```python
from build123d import *

# Parameters (mm, degrees)
SKETCH1_W            = 40.5
SKETCH1_H            = 20
BOSS_EXTRUDE1_DEPTH  = 35.5
BOSS_EXTRUDE2_DEPTH  = 2
SKETCH3_R            = 6.4
BOSS_EXTRUDE3_DEPTH  = 1
SKETCH4_R            = 5.575
BOSS_EXTRUDE4_DEPTH  = 0.5
BOSS_EXTRUDE5_DEPTH  = 2.5
MIRROR2_COPY_1_DEPTH = 2.5


with BuildPart() as part:
    # Sketch1 → Boss-Extrude1 (new body)
    with BuildSketch(Plane(origin=(0, 0, 0), x_dir=(1, 0, 0), z_dir=(0, 1, 0))):
        Rectangle(SKETCH1_W, SKETCH1_H)
    extrude(amount=BOSS_EXTRUDE1_DEPTH)

    # Sketch2 → Boss-Extrude2 (add)
    with BuildSketch(Plane(origin=(0, 35.5, 0), x_dir=(1, 0, 0), z_dir=(0, 1, 0))):
        with BuildLine():
            Line((-5.75, -9), (14.25, -9))
            Line((14.25, -9), (14.25, -4.8))
            ThreePointArc((14.25, -4.8), (16.65, 0), (14.25, 4.8))
            Line((14.25, 4.8), (14.25, 9))
            Line((14.25, 9), (-5.75, 9))
            ThreePointArc((-5.75, 9), (-20.108898944, 0), (-5.75, -9))
        make_face()
    extrude(amount=BOSS_EXTRUDE2_DEPTH)

    # Sketch3 → Boss-Extrude3 (add)
    with BuildSketch(Plane(origin=(0, 37.5, 0), x_dir=(1, 0, 0), z_dir=(0, 1, 0))):
        with Locations(Location((-10.108898944, 0, 0), (0, 0, 270))):
            Circle(SKETCH3_R)
    extrude(amount=BOSS_EXTRUDE3_DEPTH)

    # Sketch4 → Boss-Extrude4 (add)
    with BuildSketch(Plane(origin=(0, 38.5, 0), x_dir=(1, 0, 0), z_dir=(0, 1, 0))):
        with Locations(Location((-10.108898944, 0, 0), (0, 0, 270))):
            Circle(SKETCH4_R)
    extrude(amount=BOSS_EXTRUDE4_DEPTH)

    # Sketch5 → Boss-Extrude5 (add)
    with BuildSketch(Plane(origin=(0, 29.5, 0), x_dir=(1, 0, 0), z_dir=(0, 1, 0))):
        with BuildLine():
            Line((20.25, 9), (27.25, 9))
            Line((27.25, 9), (27.25, 6.25))
            Line((27.25, 6.25), (26.177050983, 6.25))
            ThreePointArc((26.177050983, 6.25), (22.25, 4.75), (26.177050983, 3.25))
            Line((26.177050983, 3.25), (27.25, 3.25))
            Line((27.25, 3.25), (27.25, 0))
            Line((27.25, 0), (20.25, 0))
            Line((20.25, 0), (20.25, 9))
        make_face()
    boss_extrude5 = extrude(amount=-BOSS_EXTRUDE5_DEPTH)

    # Mirror1: Boss-Extrude5 across plane
    add(boss_extrude5.mirror(Plane(origin=(0, 0, 0), x_dir=(0, 0, 1), z_dir=(1, 0, 0))))

    # Mirror2: Boss-Extrude5 across plane
    add(boss_extrude5.mirror(Plane.XY))

    # Mirror2 copy 1 sketch → Mirror2 copy 1 (add)
    with BuildSketch(Plane(origin=(0, 29.5, 0), x_dir=(-1, 0, 0), z_dir=(0, 1, 0))):
        with BuildLine():
            Line((20.25, 9), (27.25, 9))
            Line((27.25, 9), (27.25, 6.25))
            Line((27.25, 6.25), (26.177050983, 6.25))
            ThreePointArc((26.177050983, 6.25), (22.25, 4.75), (26.177050983, 3.25))
            Line((26.177050983, 3.25), (27.25, 3.25))
            Line((27.25, 3.25), (27.25, 0))
            Line((27.25, 0), (20.25, 0))
            Line((20.25, 0), (20.25, 9))
        make_face()
    extrude(amount=-MIRROR2_COPY_1_DEPTH)


solid = part.part
```
For this review, take the finished solid that the model builds, in its own axes (mm). A direction names the side the tool comes from. Round coordinates to 2 decimals unless told otherwise and drop trailing zeros. Write each loop counter-clockwise with the first axis right and the second up, starting at its lowest first coordinate (ties: lowest second). Pieces come first, ordered by that corner, then holes. Notation, with made-up numbers: (-3, 6.5) - (21, 6.5) arc R12 ccw to (21, 10.5) - close; hole circle Ø11 at (55.25, -29.75). An arc over 180 degrees is marked (long way). Answer as a JSON object with one key per item and string values.
1. Tool access review of faces 5 (the face through (-27, 28, -6.25)), 6 (the face through (23, 27, 0)), 7 (the face through (-20.09, 35.5, 2.18)): name each direction out of +Z, -Z, +X, -X, +Y, -Y from which nothing blocks a thin tool from reaching the whole face with its end or side.
Response values:
{"face 5": "-X, +Y, -Y", "face 6": "+Z, -Z, +X, -Y", "face 7": "-X, +Y"}
2. Draft analysis for pull direction Z (two halves, no side actions). For faces 1 (the face through (-27, 28, -3.25)), 2 (the face through (23, 29.5, 0)), 3 (the face through (-24, 28, 9)), 4 (the face through (22.25, 28.27, 4.83)), state which applies: +Z half, -Z half, draft (parallel to the pull), parting line (faces both ways), or undercut.
Response values:
{"face 1": "undercut", "face 2": "draft", "face 3": "+Z half", "face 4": "undercut"}
3. We need section A-A on x = -24.5. Give the boundary of the cut face in (y, z).
Response values:
{"outline": "(27, -9) - (29.5, -9) - (29.5, -7) - (27, -7) - close; (27, -2.5) - (29.5, -2.5) - (29.5, 2.5) - (27, 2.5) - close; (27, 7) - (29.5, 7) - (29.5, 9) - (27, 9) - close"}
4. To check wall thickness, follow line 1 along Z through (x, y) = (-24.5, 28.15); line 2 along Z through (x, y) = (21, 29); line 3 along X through (y, z) = (28.75, -4.75). State the ranges of each line that lie inside material, in increasing order.
Response values:
{"line 1": "z = -9 to -7, -2.5 to 2.5, 7 to 9", "line 2": "z = -9 to 9", "line 3": "x = -22.25 to 22.25"}
5. For pin 1 Ø3 at (x, z) = (9, -5) entering from +Y; pin 2 Ø1.6 at (y, z) = (36.5, 7.5) entering from +X; pin 3 Ø5 at (y, z) = (34.5, -6) entering from -X, all flat-tipped, find the tip position at first contact; note any pin that passes through.
Response values:
{"pin 1": "stops at y = 37.5", "pin 2": "stops at x = 14.25", "pin 3": "stops at x = -20.25"}
6. We need section B-B on x = -3. Give the boundary of the cut face in (y, z).
Response values:
{"outline": "(0, -10) - (35.5, -10) - (35.5, -9) - (37.5, -9) - (37.5, 9) - (35.5, 9) - (35.5, 10) - (0, 10) - close"}
7. We need section C-C on z = 0. Give the boundary of the cut face in (x, y).
Response values:
{"outline": "(-27.25, 27) - (-20.25, 27) - (-20.25, 0) - (20.25, 0) - (20.25, 27) - (27.25, 27) - (27.25, 29.5) - (20.25, 29.5) - (20.25, 35.5) - (16.65, 35.5) - (16.65, 37.5) - (-3.71, 37.5) - (-3.71, 38.5) - (-4.53, 38.5) - (-4.53, 39) - (-15.68, 39) - (-15.68, 38.5) - (-16.51, 38.5) - (-16.51, 37.5) - (-20.11, 37.5) - (-20.11, 35.5) - (-20.25, 35.5) - (-20.25, 29.5) - (-27.25, 29.5) - close"}
8. We need section D-D on y = 6. Give the boundary of the cut face in (x, z), then the cut area to 3 significant figures.
Response values:
{"outline": "(-20.25, -10) - (20.25, -10) - (20.25, 10) - (-20.25, 10) - close", "area": "810 mm2"}
